Here's how the part is built. I have some questions about the finished solid (model axes, mm). A direction names the side the tool comes from. Round coordinates to 2 decimals unless told otherwise and drop trailing zeros. Order: outer loops, then holes, each group sorted by start corner. A loop starts at its lowest first (then second) coordinate and runs counter-clockwise, first axis right, second up.
```python
from build123d import *

# Parameters (mm, degrees)
SKETCH_1_R               = 5
SKETCH_1_R_2             = 2.5
EXTRUDE_1_DEPTH          = 10
SKETCH_2_R               = 2.5
EXTRUDE_2_DEPTH          = 4
PATTERN_CIRCULAR_1_COUNT = 4
CUT_EXTRUDE_2_DEPTH      = 2.5
PATTERN_CIRCULAR_2_COUNT = 4
EXTRUDE_5_DEPTH          = 10
PATTERN_CIRCULAR_3_COUNT = 4


with BuildPart() as part:
    # 草图1 → 凸台-拉伸1 (new body)
    with BuildSketch(Plane.XY):
        Circle(SKETCH_1_R)
        Circle(SKETCH_1_R_2, mode=Mode.SUBTRACT)
    extrude(amount=EXTRUDE_1_DEPTH)

    # 草图2 → 凸台-拉伸2 (add, symmetric)
    with BuildSketch(Plane(origin=(0, 0, 0), x_dir=(1, 0, 0), z_dir=(0, 1, 0))):
        with BuildLine():
            Line((-5, 0), (-10, 0))
            ThreePointArc((-10, 0), (-15, -5), (-10, -10))
            Line((-10, -10), (-5, -10))
            Line((-5, -10), (-4.632725414, -10))
            Line((-4.632725414, -10), (-3.973155126, -10))
            Line((-3.973155126, -10), (-3.973155126, 0))
            Line((-3.973155126, 0), (-4.632725414, 0))
            Line((-4.632725414, 0), (-5, 0))
        make_face()
        with Locations(Location((-10, -5, 0), (0, 0, 270))):
            Circle(SKETCH_2_R, mode=Mode.SUBTRACT)
    extrude_2 = extrude(amount=EXTRUDE_2_DEPTH, both=True)

    # 阵列(圆周)1: 凸台-拉伸2 ×4 about axis
    pattern_circular_1_axis = Axis((0, 0, 0), (0, 0, 1))
    for i in range(1, PATTERN_CIRCULAR_1_COUNT):
        add(extrude_2.rotate(pattern_circular_1_axis, i * 360 / PATTERN_CIRCULAR_1_COUNT))

    # 草图4 → 切除-拉伸2 (cut, symmetric)
    with BuildSketch(Plane(origin=(0, 0, 0), x_dir=(1, 0, 0), z_dir=(0, 1, 0))):
        with BuildLine():
            Line((-10, 0), (-6, 0))
            Line((-6, 0), (-6, -10))
            Line((-6, -10), (-10, -10))
            ThreePointArc((-10, -10), (-15, -5), (-10, 0))
        make_face()
    cut_extrude_2 = extrude(amount=CUT_EXTRUDE_2_DEPTH, both=True, mode=Mode.SUBTRACT)

    # 阵列(圆周)2: 切除-拉伸2 ×4 about axis
    pattern_circular_2_axis = Axis((0, 0, 0), (0, 0, 1))
    for i in range(1, PATTERN_CIRCULAR_2_COUNT):
        add(cut_extrude_2.rotate(pattern_circular_2_axis, i * 360 / PATTERN_CIRCULAR_2_COUNT), mode=Mode.SUBTRACT)

    # 草图5 → 凸台-拉伸5 (add)
    with BuildSketch(Plane(origin=(0, 0, 0), x_dir=(-1, 0, 0), z_dir=(0, 0, -1))):
        Polygon((-3.973155126, 3.973155126), (-3.035463449, 3.973155126), (-3.973155126, 3.035463449), align=None)
    extrude_5 = extrude(amount=-EXTRUDE_5_DEPTH)

    # 阵列(圆周)3: 凸台-拉伸5 ×4 about axis
    pattern_circular_3_axis = Axis((0, 0, 0), (0, 0, -1))
    for i in range(1, PATTERN_CIRCULAR_3_COUNT):
        add(extrude_5.rotate(pattern_circular_3_axis, i * 360 / PATTERN_CIRCULAR_3_COUNT))


solid = part.part
```
1) I need wall thicknesses on line 1 (Y direction, x = 3.1, z = 5); line 2 (X direction, y = -12.5, z = 0.75); line 3 (Y direction, x = 0, z = 2). Which ranges of each line are inside material? Lowest first, please.
2) If we section it at B-B (y = 7): Write out the boundary of the cut face in (x, z).
3) We'd pull the mould along X, two halves only. Please class faces 5 (the flat face through (6, 0, 5)), 6 (the flat face through (-7, 4, 5)), 7 (the flat face through (2.5, -11.4, 2.7)): +X half, -X half, draft (parallel to the pull), parting line (faces both ways), or undercut.
4) If we section it at C-C (x = -8.5): Write out the boundary of the cut face in (y, z).
5) For faces 1 (the flat face through (-2.5, 11.4, 2.7)), 2 (the flat face through (7, -4, 5)), 3 (the flat face through (0, -6, 5)), 4 (the flat face through (-11.4, 2.5, 2.7)), which set-ups out of +Z, -Z, +X, -X, +Y, -Y let a thin tool reach every point of the face, with its end or its side?
6) If we section it at A-A (x = 0): Write out the boundary of the cut face in (y, z), plus the area to 3 significant figures.
7) I'm going to push flat-ended pins straight in: pin 1 (6 mm diameter, centred on x = -10, z = 5, fed in from +Y); pin 2 (6.5 mm diameter, centred on x = 0, y = 0, fed in from +Z); pin 3 (1.5 mm diameter, centred on x = 2.5, y = 12, fed in from +Z); pin 4 (3 mm diameter, centred on y = -7, z = 5.5, fed in from +X). Where does each tip first touch, or does it pass through?
Solutions:
1. line 1: y = -15 to -12.5, -7.5 to 7.5, 12.5 to 15
1. line 2: x = -4 to -2.5, 2.5 to 4
1. line 3: y = -6 to -2.5, 2.5 to 6
2. outline: (-4, 0) - (-2.5, 0) - (-2.5, 10) - (-4, 10) - close; (2.5, 0) - (4, 0) - (4, 10) - (2.5, 10) - close
3. face 5: +X half
3. face 6: draft
3. face 7: undercut
4. outline: (-4, 0) - (-2.5, 0) - (-2.5, 3) - (-4, 3) - close; (-4, 7) - (-2.5, 7) - (-2.5, 10) - (-4, 10) - close; (2.5, 0) - (4, 0) - (4, 3) - (2.5, 3) - close; (2.5, 7) - (4, 7) - (4, 10) - (2.5, 10) - close
5. face 1: +Z, -Z, +Y
5. face 2: +Z, -Z, +X, -Y
5. face 3: +Z, -Z, -Y
5. face 4: +Z, -Z, -X
6. outline: (-6, 0) - (-2.5, 0) - (-2.5, 10) - (-6, 10) - close; (2.5, 0) - (6, 0) - (6, 10) - (2.5, 10) - close
6. area: 70.0 mm2
7. pin 1: stops at y = 4
7. pin 2: stops at z = 10
7. pin 3: stops at z = 9.84
7. pin 4: stops at x = 4
